Check sheet for the modelled part. Datum: model origin and axes. Units: mm. Face numbers are marked on the shaded views. Round coordinates to 2 decimals unless told otherwise and drop trailing zeros. Order: outer loops, then holes, each group sorted by start corner. A loop starts at its lowest first (then second) coordinate and runs counter-clockwise, first axis right, second up. Notation, with made-up numbers: (-26.5, 22) -> (12.5, 22) arc R30 ccw to (12.5, 46) -> close; hole circle Ø9 at (-31, 3.5). An arc over 180 degrees is marked (long way). Answer in a Markdown table with one row per item.
from build123d import *

# Parameters (mm, degrees)
SKETCH_1_R      = 1
EXTRUDE_1_DEPTH = 1.5
FILLET_1_R      = 1


with BuildPart() as part:
    # 草图1 → 凸台-拉伸1 (new body)
    with BuildSketch(Plane.XY):
        Polygon((64.3, -0.39974336), (59.3, -0.39974336), (59.3, 3.10025664), (60, 3.10025664), (60, 4.60025664), (55.6, 4.60025664), (55.6, 3.10025664), (57.8, 3.10025664), (57.8, -0.39974336), (52.8, -0.39974336), (52.8, 4.60025664), (2.8, 4.60025664), (2.8, -0.39974336), (-2.2, -0.39974336), (-2.2, 3.10025664), (0, 3.10025664), (0, 4.60025664), (-4.42519, 4.60025664), (-4.42519, 3.10025664), (-3.75, 3.10025664), (-3.75, -0.39974336), (-8.75, -0.39974336), (-8.75, 8.60025664), (-0.803608582, 8.60025664), (16.62882385, 30.10025664), (34.845120873, 30.10025664), (49.819650388, 30.10025664), (64.3, 12.241158786), align=None)
        with Locations((33.25, 27.10025664)):
            Circle(SKETCH_1_R, mode=Mode.SUBTRACT)
        with Locations((48.25, 8.60025664)):
            Circle(SKETCH_1_R, mode=Mode.SUBTRACT)
        with Locations((18.25, 8.60025664)):
            Circle(SKETCH_1_R, mode=Mode.SUBTRACT)
        with Locations((58.525, 14.60025664)):
            Circle(SKETCH_1_R, mode=Mode.SUBTRACT)
        with Locations(Location((7.975, 14.60025664, 0), (0, 0, 180))):
            Circle(SKETCH_1_R, mode=Mode.SUBTRACT)
        Polygon((59.527646909, 8.60025664), (52.112217956, 8.60025664), (37.112217956, 27.10025664), (44.527646909, 27.10025664), align=None, mode=Mode.SUBTRACT)
        Polygon((44.387782044, 8.60025664), (33.25, 22.336854495), (22.112217956, 8.60025664), align=None, mode=Mode.SUBTRACT)
        Polygon((21.972353091, 27.10025664), (29.387782044, 27.10025664), (14.387782044, 8.60025664), (6.972353091, 8.60025664), align=None, mode=Mode.SUBTRACT)
    extrude(amount=EXTRUDE_1_DEPTH)

    # 圆角1
    fillet_1_edges = [part.edges().sort_by_distance(p)[0] for p in [
        (64.3, -0.39974336, 0.75),
        (52.8, -0.39974336, 0.75),
        (2.8, -0.39974336, 0.75),
        (-8.75, -0.39974336, 0.75),
        (-8.75, 8.60025664, 0.75),
        (-0.803608582, 8.60025664, 0.75),
        (16.62882385, 30.10025664, 0.75),
        (49.819650388, 30.10025664, 0.75),
        (64.3, 12.241158786, 0.75),
    ]]
    fillet(fillet_1_edges, radius=FILLET_1_R)


solid = part.part
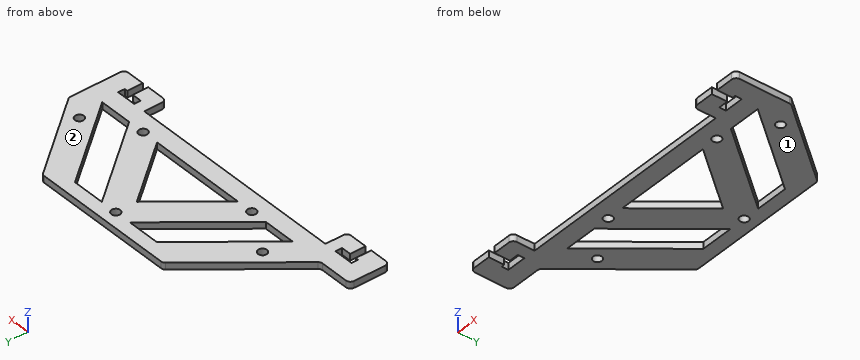
Item 1: Cross-section at A-A (y = 23). Record the boundary of the cut face in (x, z), and give its area (3 significant figures).
Result sheet:
| item | result |
|---|---|
| outline | (10.87, 0) -> (18.65, 0) -> (18.65, 1.5) -> (10.87, 1.5) -> close; (26.06, 0) -> (40.44, 0) -> (40.44, 1.5) -> (26.06, 1.5) -> close; (47.85, 0) -> (55.58, 0) -> (55.58, 1.5) -> (47.85, 1.5) -> close |
| area | 44.8 mm^2 |
Item 2: Cross-section at C-C (x = 10). Record the boundary of the cut face in (y, z).
Result sheet:
| item | result |
|---|---|
| outline | (4.6, 0) -> (8.6, 0) -> (8.6, 1.5) -> (4.6, 1.5) -> close; (12.33, 0) -> (21.92, 0) -> (21.92, 1.5) -> (12.33, 1.5) -> close |
Item 3: Scan lines: line 1 (X direction, y = 3, z = 1.4); line 2 (Y direction, x = -1.5, z = 1.35); line 3 (X direction, y = 11, z = 0.55). Record each from-to range of solid material in increasing order. Write a range as [from, to].
Result sheet:
| item | result |
|---|---|
| line 1 | x = [-8.75, -3.75], [-2.2, 2.8], [52.8, 57.8], [59.3, 64.3] |
| line 2 | y = [-0.4, 3.1], [4.6, 8.6] |
| line 3 | x = [1.14, 8.92], [16.33, 24.06], [42.44, 50.17], [57.58, 64.3] |
Item 4: Cross-section at B-B (x = 18.25). Record the boundary of the cut face in (y, z), and give its area (3 significant figures).
Result sheet:
| item | result |
|---|---|
| outline | (4.6, 0) -> (7.6, 0) -> (7.6, 1.5) -> (4.6, 1.5) -> close; (9.6, 0) -> (13.36, 0) -> (13.36, 1.5) -> (9.6, 1.5) -> close; (22.51, 0) -> (30.1, 0) -> (30.1, 1.5) -> (22.51, 1.5) -> close |
| area | 21.5 mm^2 |
Item 5: Mould release check, pull along Z, two halves, no side actions. Record for the marked faces 1 and 2: pulls with the +Z half, pulls with the -Z half, needs draft (parallel to the pull), parting line crosses it, or undercut.
Result sheet:
| item | result |
|---|---|
| face 1 | pulls with the -Z half |
| face 2 | pulls with the +Z half |
Item 6: Cross-section at D-D (z = 1.2). State how many separate pieces and enclosed holes the cut face has, and give its area (3 significant figures).
Result sheet:
| item | result |
|---|---|
| separate pieces | 1 |
| enclosed holes | 8 |
| area | 1,020 mm^2 |
Item 7: Depth check by flat-ended pin: P1, Ø0.5, axis at x = -4, z = 1, coming from the +Y side; P2, Ø0.8, axis at x = 35.5, z = 1, coming from the -Y side. Enter the tip coordinate at first touch or a pass-through.
Result sheet:
| item | result |
|---|---|
| P1 | stops at y = 8.6 |
| P2 | stops at y = 4.6 |
